from build123d import *

# Parameters (mm, degrees)
VERRUNDUNG1_R = 0.5


with BuildPart() as part:
    # Skizze1 → Rotation1 (revolve)
    with BuildSketch(Plane.XY):
        Polygon((-78.778077973, 1.754378812), (-78.778077973, 6.754378812), (-51.778077973, 6.754378812), (-51.778077973, 7.754378812), (-36.078077973, 7.754378812), (-36.078077973, 6.754378812), (-26.078077973, 6.754378812), (-25.078077973, 6.754378812), (-20.078077973, 6.754378812), (-20.078077973, 1.754378812), align=None)
    revolve(axis=Axis((-20.078077973, 1.754378812, 0), (-1, 0, 0)))

    # Verrundung1
    verrundung1_edges = [part.edges().sort_by_distance(p)[0] for p in [
        (-78.778077973, -3.245621188, 0),
        (-20.078077973, -3.245621188, 0),
    ]]
    fillet(verrundung1_edges, radius=VERRUNDUNG1_R)


solid = part.part
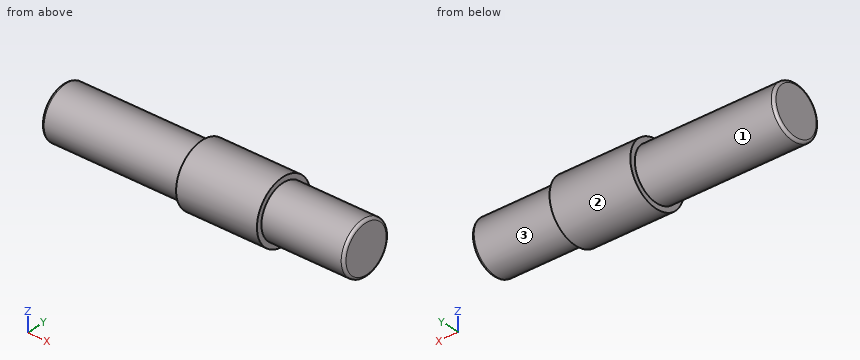
Read the model definition and answer for the solid it produces. Units are mm, in the model's axes. Face numbers are marked on the shaded views. A direction names the side the tool comes from. Give positions to 0.01 mm unless a question says otherwise; leave off trailing zeros. Write each loop counter-clockwise with the first axis right and the second up, starting at its lowest first coordinate (ties: lowest second). Pieces come first, ordered by that corner, then holes. Notation, with made-up numbers: (38.25, -25) - (84.25, -25) arc R20 cw to (84.25, -14) - close; hole circle Ø11 at (12.25, 83.5). An arc over 180 degrees is marked (long way). Return JSON: item names as keys, results as strings.
Q1. A cutting plane is placed at B-B, the plane x = -42. Determine the outline of the cut face in (y, z), and give its area (3 significant figures).
Reply:
{"outline": "circle Ø12 at (1.75, 0)", "area": "113 mm²"}
Q2. Consider line 1 along X through (y, z) = (-3.25, 1.25); line 2 along Y through (x, z) = (-47.5, -4.25); line 3 along Z through (x, y) = (-59, -1). Determine where each line is inside the solid, lowest interval first. Write a range as [from, to].
Reply:
{"line 1": "[-51.78, -36.08]", "line 2": "[-2.48, 5.99]", "line 3": "[-4.17, 4.17]"}
Q3. A cutting plane is placed at C-C, the plane x = -54. Determine the outline of the cut face in (y, z), and give its area (3 significant figures).
Reply:
{"outline": "circle Ø10 at (1.75, 0)", "area": "78.5 mm²"}
Q4. For the marked faces 1, 2 and 3, determine the directions among +Z, -Z, +X, -X, +Y, -Y from which every point of the face is accessible in a straight line to the end or side of a thin tool.
Reply:
{"face 1": "-X", "face 2": "+X, -X", "face 3": "+X"}
Q5. A cutting plane is placed at A-A, the plane z = 0. Determine the outline of the cut face in (x, y), and give its area (3 significant figures).
Reply:
{"outline": "(-78.78, -2.75) arc R0.5 ccw to (-78.28, -3.25) - (-51.78, -3.25) - (-51.78, -4.25) - (-36.08, -4.25) - (-36.08, -3.25) - (-20.58, -3.25) arc R0.5 ccw to (-20.08, -2.75) - (-20.08, 6.25) arc R0.5 ccw to (-20.58, 6.75) - (-36.08, 6.75) - (-36.08, 7.75) - (-51.78, 7.75) - (-51.78, 6.75) - (-78.28, 6.75) arc R0.5 ccw to (-78.78, 6.25) - close", "area": "618 mm²"}
Q6. Given P1, Ø2, axis at x = -57, y = 0, coming from the -Z side; P2, Ø1.5, axis at x = -42.5, y = 1.5, coming from the -Z side; P3, Ø1, axis at x = -27, y = 6.5, coming from the -Z side; P4, Ø2, axis at x = -26, y = -3, coming from the +Z side, each flat-ended and moving along its own axis, determine where each tip first touches the part or whether it passes through.
Reply:
{"P1": "z = -4.94", "P2": "z = -6", "P3": "z = -2.64", "P4": "z = 3.3"}
